from build123d import *

# Parameters (mm, degrees)
F0_W     = 50
F0_H     = 50
F1_DEPTH = 15
F3_DEPTH = 10
F5_DEPTH = 5
F6_W     = 30
F6_H     = 5.4
F7_DEPTH = 30


with BuildPart() as f1:
    # F0 (on Top) → F1 (new body)
    with BuildSketch(Plane.XY):
        with Locations((25, -25)):
            Rectangle(F0_W, F0_H)
    extrude(amount=F1_DEPTH)

    # F2 (on face) → F3 (join)
    with BuildSketch(Plane.XY.offset(15)):
        Polygon((15, -30), (15, -50), (35, -50), (35, -30), (25, -17.510004), align=None)
    extrude(amount=F3_DEPTH)

    # F4 (on face) → F5 (cut)
    with BuildSketch(Plane(origin=(0, 0, 0), x_dir=(1, 0, 0), z_dir=(0, 0, -1))):
        Polygon((35, 50), (15, 50), (15, 30), (25, 17.510004), (35, 30), align=None)
    extrude(amount=-F5_DEPTH, mode=Mode.SUBTRACT)

    # F6 (on face) → F7 (cut)
    with BuildSketch(Plane.YZ.offset(50)):
        with Locations((-15, 7.7)):
            Rectangle(F6_W, F6_H)
    extrude(amount=-F7_DEPTH, mode=Mode.SUBTRACT)


solid = f1.part
Part model, mm, in its own coordinate system. A direction names the side the tool comes from. Give positions to 0.01 mm unless a question says otherwise; leave off trailing zeros. Write each loop counter-clockwise with the first axis right and the second up, starting at its lowest first coordinate (ties: lowest second). Pieces come first, ordered by that corner, then holes.
1) Pin check, flat tips, straight feed: pin 1 (2.5 mm diameter, centred on x = 42.5, z = 7, fed in from +Y); pin 2 (4 mm diameter, centred on x = 15.5, z = 17.5, fed in from +Y); pin 3 (2.5 mm diameter, centred on y = -18, z = 7, fed in from +X). Stop position of each tip, or through.
Resolved:
pin 1: stops at y = -30
pin 2: stops at y = -26.88
pin 3: stops at x = 20
2) Cut at B-B on x = 29.5. Write the cut outline in (y, z).
Resolved:
outline: (-50, 5) - (-30, 5) - (-30, 10.4) - (0, 10.4) - (0, 15) - (-23.13, 15) - (-23.13, 25) - (-50, 25) - close; (-23.13, 0) - (0, 0) - (0, 5) - (-23.13, 5) - close
3) Probe L1, parallel to Z at x = 46, y = -21; L2, parallel to Z at x = 12.5, y = -6; L3, parallel to Z at x = 20.5, y = -46. List the from-to ranges inside material, lowest first.
Resolved:
L1: z = 0 to 5, 10.4 to 15
L2: z = 0 to 15
L3: z = 5 to 25
4) Cut at A-A on y = -29. Write the cut outline in (x, z), then the cut area to 3 significant figures.
Resolved:
outline: (0, 0) - (15.8, 0) - (15.8, 5) - (20, 5) - (20, 10.4) - (50, 10.4) - (50, 15) - (34.2, 15) - (34.2, 25) - (15.8, 25) - (15.8, 15) - (0, 15) - close; (34.2, 0) - (50, 0) - (50, 5) - (34.2, 5) - close
area: 680 mm2
5) Which spindle directions (+Z, -Z, +X, -X, +Y, -Y) get a long thin tool onto all of the face, cutting with end or side? Do faces 5 (the face through (30.07, -23.84, 19.93)), 6 (the face through (29.93, -23.67, 2.46)), 7 (the face through (20.07, -23.67, 19.93)). Say none if no direction does.
Resolved:
face 5: +Z, +X, +Y
face 6: -Z, -Y
face 7: +Z, -X, +Y
6) Cut at C-C on x = 42. Write the cut outline in (y, z), then the cut area to 3 significant figures.
Resolved:
outline: (-50, 0) - (0, 0) - (0, 5) - (-30, 5) - (-30, 10.4) - (0, 10.4) - (0, 15) - (-50, 15) - close
area: 588 mm2
7) Two-plate mould, pull along Z, no slides. Class faces 1 (the face through (35, -15, 5)), 2 (the face through (35, -30, 8)), 3 (the face through (19.93, -23.84, 2.46)), 4 (the face through (25, -40, 5)): released by +Z, released by -Z, zero draft, split by the parting line, or undercut.
Resolved:
face 1: undercut
face 2: undercut
face 3: zero draft
face 4: released by -Z
8) Cut at D-D on z = 9.75. Write the cut outline in (x, y), then the cut area to 3 significant figures.
Resolved:
outline: (0, -50) - (50, -50) - (50, -30) - (20, -30) - (20, 0) - (0, 0) - close
area: 1,600 mm2
